The listing builds one solid part. Answer for the finished solid, in the listing's coordinates (mm). A direction names the side the tool comes from. Give positions to 0.01 mm unless a question says otherwise; leave off trailing zeros. Write each loop counter-clockwise with the first axis right and the second up, starting at its lowest first coordinate (ties: lowest second). Pieces come first, ordered by that corner, then holes. Notation, with made-up numbers: (62, 23) -> (81, 23) arc R13 ccw to (81, 47) -> close; hole circle Ø4 at (70.5, 55.25). An arc over 180 degrees is marked (long way). Put each result on its own line as item: value. Start each with the question number.
1) A cutting plane is placed at D-D (x = 10.25). Write down the section's boundary in (y, z), then the cut area to 3 significant figures.
2) For faces 1 (the flat face through (9.25, 0, -9)), 2 (the flat face through (0, -10, -4.064)), 3 (the flat face through (-10, 0, -4.064)), determine the directions among +Z, -Z, +X, -X, +Y, -Y from which every point of the face is accessible in a straight line to the end or side of a thin tool.
3) Flat-ended cylindrical pins translate along their axes: pin 1 Ø8.5 at (x, z) = (3.5, -8.5) entering from -Y; pin 2 Ø5 at (x, z) = (5, -8.5) entering from +Y; pin 3 Ø5 at (y, z) = (-3, -7) entering from +X. Find the tip coordinate at first contact, or state that the pin passes through.
4) For a pull along Z with two mould halves and no side action, classify faces 4 (the flat face through (0, 10, -4.064)), 5 (the flat face through (0, 0, -17.018)), 6 (the flat face through (0, 0, 0)) as released by +Z, released by -Z, zero draft, split by the parting line, or undercut.
5) A cutting plane is placed at A-A (x = 0). Write down the section's boundary in (y, z) (3 decimals).
6) Find the intervals of material crossed by line 1 along Z through (x, y) = (-10, -6); line 2 along Y through (x, z) = (4.25, -9), in increasing order. Write a range as from..to.
7) A cutting plane is placed at C-C (z = -5.75). Write down the section's boundary in (x, y) (3 decimals).
from build123d import *
from build123d.topology import SkipClean

# Parameters (mm, degrees)
SKETCH1_R           = 11.975000032
BOSS_EXTRUDE1_DEPTH = 4.064
BOSS_EXTRUDE2_DEPTH = 10.414
SKETCH3_R           = 11.975000032
BOSS_EXTRUDE3_DEPTH = 2.54


with BuildPart() as part:
    # Sketch1 → Boss-Extrude1 (new body)
    with BuildSketch(Plane.XY):
        Circle(SKETCH1_R)
    extrude(amount=-BOSS_EXTRUDE1_DEPTH)

    # Sketch2 → Boss-Extrude2 (add)
    with SkipClean():  # the faces are left unmerged after this step: merging them gives an invalid solid
        with BuildSketch(Plane(origin=(0, 0, -4.064), x_dir=(-1, 0, 0), z_dir=(0, 0, -1))):
            with BuildLine():
                ThreePointArc((9.250000032, 7.605138077), (8.467603727, 8.467603727), (7.605138077, 9.250000032))
                Line((7.605138077, 9.250000032), (-7.605138077, 9.250000032))
                ThreePointArc((-7.605138077, 9.250000032), (-8.467603727, 8.467603727), (-9.250000032, 7.605138077))
                Line((-9.250000032, 7.605138077), (-9.250000032, -7.605138077))
                ThreePointArc((-9.250000032, -7.605138077), (-8.467603727, -8.467603727), (-7.605138077, -9.250000032))
                Line((-7.605138077, -9.250000032), (7.605138077, -9.250000032))
                ThreePointArc((7.605138077, -9.250000032), (8.467603727, -8.467603727), (9.250000032, -7.605138077))
                Line((9.250000032, -7.605138077), (9.250000032, 7.605138077))
            make_face()
        extrude(amount=BOSS_EXTRUDE2_DEPTH)

    # Sketch3 → Boss-Extrude3 (add)
    with BuildSketch(Plane(origin=(0, 0, -14.478), x_dir=(-1, 0, 0), z_dir=(0, 0, -1))):
        with Locations(Location((0, 0, 0), (0, 0, 180))):
            Circle(SKETCH3_R)
    extrude(amount=BOSS_EXTRUDE3_DEPTH)


solid = part.part
Reply:
1. outline: (-6.19, -17.02) -> (6.19, -17.02) -> (6.19, -14.48) -> (-6.19, -14.48) -> close; (-6.19, -4.06) -> (6.19, -4.06) -> (6.19, 0) -> (-6.19, 0) -> close
1. area: 81.8 mm2
2. face 1: +X, +Y, -Y
2. face 2: +X, -X, -Y
2. face 3: -X, +Y, -Y
3. pin 1: stops at y = -9.25
3. pin 2: stops at y = 9.25
3. pin 3: stops at x = 9.25
4. face 4: undercut
4. face 5: released by -Z
4. face 6: released by +Z
5. outline: (-11.975, -17.018) -> (11.975, -17.018) -> (11.975, -14.478) -> (9.25, -14.478) -> (9.25, -4.064) -> (11.975, -4.064) -> (11.975, 0) -> (-11.975, 0) -> (-11.975, -4.064) -> (-9.25, -4.064) -> (-9.25, -14.478) -> (-11.975, -14.478) -> close
6. line 1: z = -17.02..-14.48, -4.06..0
6. line 2: y = -9.25..9.25
7. outline: (-9.25, -7.605) arc R11.975 ccw to (-7.605, -9.25) -> (7.605, -9.25) arc R11.975 ccw to (9.25, -7.605) -> (9.25, 7.605) arc R11.975 ccw to (7.605, 9.25) -> (-7.605, 9.25) arc R11.975 ccw to (-9.25, 7.605) -> close
